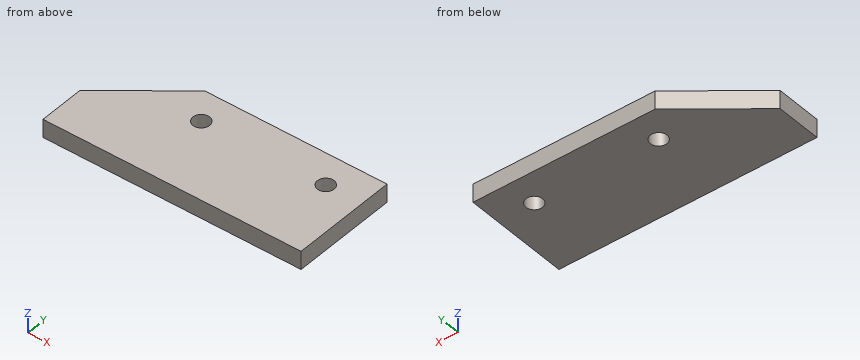
Autodesk Fusion 360 part; units mm, degrees
sketch "Z Endswitch plate" plane through (0, 0, 0) normal (0, 0, 1) x (1, 0, 0)
  line L0 (18, -15) -> (18, 20)
  circle A0 centre (6, 9.9027) radius 2.75
  line L1 (-67, 20) -> (-67, -15)
  line L2 (-67, -15) -> (18, -15)
  line L3 (-42, 20) -> (-67, 0)
  circle A1 centre (-35, 9.9027) radius 2.75
  line L4 (18, 20) -> (-67, 20)
  line L5 (18, 9.9027) -> (-67, 9.9027) construction
  dimension "d2" = 85
  dimension "d3" = 5.5
  dimension "d4" = 5.5
  dimension "d7" = 25
  dimension "d8" = 20
  dimension "d9" = 15
  dimension "d10" = 18
  dimension "d11" = 6
  dimension "d12" = 35
extrude "Extrude1" add sketch "Z Endswitch plate" along normal blind 6 contours L0 L1 L2 L3 L4
Geometry check sheet. Reference: the model listing, model coordinates, mm. Give positions to 0.01 mm unless a question says otherwise; leave off trailing zeros. Write each loop counter-clockwise with the first axis right and the second up, starting at its lowest first coordinate (ties: lowest second). Pieces come first, ordered by that corner, then holes. Notation, with made-up numbers: (71.25, 18.25) - (106.25, 18.25) arc R27 ccw to (106.25, 51.25) - close; hole circle Ø6 at (67, -8.75). An arc over 180 degrees is marked (long way). Use a Markdown table: item, result.
Q1. Section check C-C, the plane z = 2.3. Enter the section's corners in (x, y), then the cut area to 3 significant figures.
Computed:
| item | result |
|---|---|
| outline | (-67, -15) - (18, -15) - (18, 20) - (-42, 20) - (-67, 0) - close; hole circle Ø5.5 at (-35, 9.9); hole circle Ø5.5 at (6, 9.9) |
| area | 2,680 mm² |
Q2. Section check B-B, the plane y = 8. Enter the section's corners in (x, z), then the cut area to 3 significant figures.
Computed:
| item | result |
|---|---|
| outline | (-57, 0) - (-36.99, 0) - (-36.99, 6) - (-57, 6) - close; (-33.01, 0) - (4.01, 0) - (4.01, 6) - (-33.01, 6) - close; (7.99, 0) - (18, 0) - (18, 6) - (7.99, 6) - close |
| area | 402 mm² |
Q3. Section check D-D, the plane x = -44. Enter the section's corners in (y, z), then the cut area to 3 significant figures.
Computed:
| item | result |
|---|---|
| outline | (-15, 0) - (18.4, 0) - (18.4, 6) - (-15, 6) - close |
| area | 200 mm² |
Q4. Thickness scan on L1, parallel to Y at x = -35, z = 4.15; L2, parallel to Y at x = 4, z = 3.15; L3, parallel to X at y = 12, z = 3.85. Record the ranges inside material, lowest first. Write a range as [from, to].
Computed:
| item | result |
|---|---|
| L1 | y = [-15, 7.15], [12.65, 20] |
| L2 | y = [-15, 8.02], [11.79, 20] |
| L3 | x = [-52, -36.78], [-33.22, 4.22], [7.78, 18] |
Q5. Go/stop test with flat-tipped pins: P1, Ø1, axis at y = 5.5, z = 1.5, coming from the -X side; P2, Ø3, axis at x = -50.5, z = 2.5, coming from the +Y side; P3, Ø1.5, axis at x = -48, z = 2, coming from the +Y side. Record where each tip stops, or that it passes through.
Computed:
| item | result |
|---|---|
| P1 | stops at x = -60.75 |
| P2 | stops at y = 14.4 |
| P3 | stops at y = 15.8 |
Q6. Section check A-A, the plane x = 6. Enter the section's corners in (y, z).
Computed:
| item | result |
|---|---|
| outline | (-15, 0) - (7.15, 0) - (7.15, 6) - (-15, 6) - close; (12.65, 0) - (20, 0) - (20, 6) - (12.65, 6) - close |
